Model file for the job. Use its own axes, mm. Give positions to 0.01 mm unless a question says otherwise; leave off trailing zeros. Loops run counter-clockwise (first coordinate to the right, second up) from the corner with the lowest first, then second, coordinate; pieces in that order, holes last. Notation, with made-up numbers: (51, 48) - (103, 48) arc R10 cw to (103, 55) - close; hole circle Ø2 at (39, 53). An arc over 180 degrees is marked (long way). Use a Markdown table: item, result.
from build123d import *

# Parameters (mm, degrees)
SKETCH1_W           = 136
SKETCH1_H           = 50
BOSS_EXTRUDE1_DEPTH = 5
SKETCH2_W           = 24.7
SKETCH2_H           = 5
BOSS_EXTRUDE2_DEPTH = 5
SKETCH3_W           = 24.7
SKETCH3_H           = 5
BOSS_EXTRUDE3_DEPTH = 5
SKETCH4_W           = 5
SKETCH4_H           = 25
CUT_EXTRUDE1_DEPTH  = 5


with BuildPart() as part:
    # Sketch1 → Boss-Extrude1 (new body)
    with BuildSketch(Plane.XY):
        with Locations((0, 25)):
            Rectangle(SKETCH1_W, SKETCH1_H)
    extrude(amount=BOSS_EXTRUDE1_DEPTH)

    # Sketch2 → Boss-Extrude2 (add)
    with BuildSketch(Plane(origin=(0, 50, 0), x_dir=(1, 0, 0), z_dir=(0, 1, 0))):
        with Locations((-55.65, -2.5)):
            Rectangle(SKETCH2_W, SKETCH2_H)
        with Locations((55.65, -2.5)):
            Rectangle(SKETCH2_W, SKETCH2_H)
    extrude(amount=BOSS_EXTRUDE2_DEPTH)

    # Sketch3 → Boss-Extrude3 (add)
    with BuildSketch(Plane.XZ):
        with Locations((-55.65, 2.5)):
            Rectangle(SKETCH3_W, SKETCH3_H)
        with Locations((55.65, 2.5)):
            Rectangle(SKETCH3_W, SKETCH3_H)
    extrude(amount=BOSS_EXTRUDE3_DEPTH)

    # Sketch4 → Cut-Extrude1 (cut)
    with BuildSketch(Plane.XY.offset(5)):
        with Locations((0, 27.5)):
            Rectangle(SKETCH4_W, SKETCH4_H)
    extrude(amount=-CUT_EXTRUDE1_DEPTH, mode=Mode.SUBTRACT)


solid = part.part
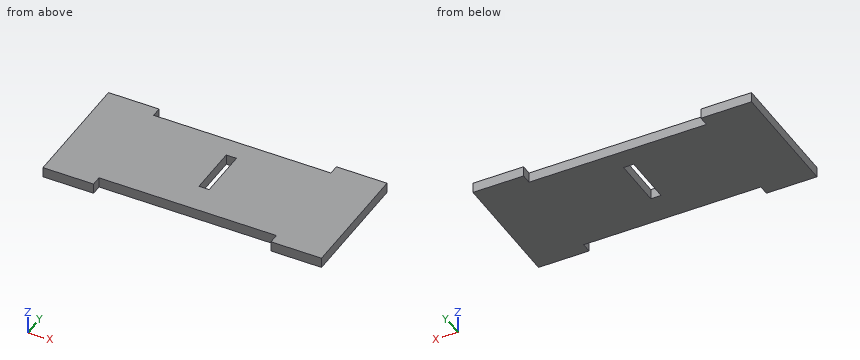
(1) Pin check, flat tip, straight feed: P1, Ø1.5, axis at x = 1, z = 2, coming from the +Y side. Stop position of the tip, or through.
Computed:
| item | result |
|---|---|
| P1 | y = 50 |
(2) Slice it at A-A, the plane y = 22. Write the cut outline in (x, z), plus the area to 3 significant figures.
Computed:
| item | result |
|---|---|
| outline | (-68, 0) - (-2.5, 0) - (-2.5, 5) - (-68, 5) - close; (2.5, 0) - (68, 0) - (68, 5) - (2.5, 5) - close |
| area | 655 mm² |
(3) Slice it at B-B, the plane z = 0.95. Write the cut outline in (x, y), plus the area to 3 significant figures.
Computed:
| item | result |
|---|---|
| outline | (-68, -5) - (-43.3, -5) - (-43.3, 0) - (43.3, 0) - (43.3, -5) - (68, -5) - (68, 55) - (43.3, 55) - (43.3, 50) - (-43.3, 50) - (-43.3, 55) - (-68, 55) - close; hole (-2.5, 15) - (2.5, 15) - (2.5, 40) - (-2.5, 40) - close |
| area | 7,170 mm² |
(4) Slice it at C-C, the plane x = 28. Write the cut outline in (y, z).
Computed:
| item | result |
|---|---|
| outline | (0, 0) - (50, 0) - (50, 5) - (0, 5) - close |
(5) Drill centre lines: probe 1 along X at (y, z) = (29.5, 2.6); probe 2 along X at (y, z) = (-1, 3.7); probe 3 along Y at (x, z) = (-1.5, 3.8). Where is each one in solid material? Low to high. Write a range as [from, to].
Computed:
| item | result |
|---|---|
| probe 1 | [-68, -2.5], [2.5, 68] |
| probe 2 | [-68, -43.3], [43.3, 68] |
| probe 3 | [0, 15], [40, 50] |
